Geometry check sheet. Reference: the model listing, model coordinates, mm. Round coordinates to 2 decimals unless told otherwise and drop trailing zeros. Loops run counter-clockwise (first coordinate to the right, second up) from the corner with the lowest first, then second, coordinate; pieces in that order, holes last. Notation, with made-up numbers: M 72.5,44 L 104.5,44 A13 cw 104.5,52 Z; hole C -22.5,38 d10. An arc over 180 degrees is marked long. Write item = value, one per line.
from build123d import *

# Parameters (mm, degrees)
SKETCH1_R           = 1.651
SKETCH1_R_2         = 2.286
BOSS_EXTRUDE1_DEPTH = 3.1496


with BuildPart() as part:
    # Sketch1 → Boss-Extrude1 (new body)
    with BuildSketch(Plane(origin=(0, 0, 0), x_dir=(1, 0, 0), z_dir=(0, 1, 0))):
        with BuildLine():
            Line((23.368, -25.4), (38.1, -10.668))
            Line((38.1, -10.668), (38.1, 10.668))
            Line((38.1, 10.668), (23.368, 25.4))
            Line((23.368, 25.4), (10.899655632, 25.4))
            ThreePointArc((10.899655632, 25.4), (0, 14.500344368), (-10.899655632, 25.4))
            Line((-10.899655632, 25.4), (-23.368, 25.4))
            Line((-23.368, 25.4), (-38.1, 10.668))
            Line((-38.1, 10.668), (-38.1, -10.668))
            Line((-38.1, -10.668), (-23.368, -25.4))
            Line((-23.368, -25.4), (-10.899655632, -25.4))
            ThreePointArc((-10.899655632, -25.4), (0, -14.500344368), (10.899655632, -25.4))
            Line((10.899655632, -25.4), (23.368, -25.4))
        make_face()
        with Locations(Location((-22.225, 19.05, 0), (0, 0, 270))):
            Circle(SKETCH1_R, mode=Mode.SUBTRACT)
        with Locations(Location((22.225, 19.05, 0), (0, 0, 270))):
            Circle(SKETCH1_R, mode=Mode.SUBTRACT)
        with Locations(Location((22.225, -19.05, 0), (0, 0, 270))):
            Circle(SKETCH1_R, mode=Mode.SUBTRACT)
        with Locations(Location((-22.225, -19.05, 0), (0, 0, 270))):
            Circle(SKETCH1_R, mode=Mode.SUBTRACT)
        with Locations(Location((9.271, -5.5118, 0), (0, 0, 270))):
            Circle(SKETCH1_R_2, mode=Mode.SUBTRACT)
        with Locations(Location((21.971, 5.5118, 0), (0, 0, 270))):
            Circle(SKETCH1_R_2, mode=Mode.SUBTRACT)
    extrude(amount=BOSS_EXTRUDE1_DEPTH)


solid = part.part
(1) Release check for a two-part mould opening along Z. For faces 1 (the cylindrical face through (-21.11, 1.55, -20.27)), 2 (the flat face through (-30.63, 1.55, -18.14)), 3 (the flat face through (-30.84, 1.55, 17.93)) record: released by +Z, released by -Z, zero draft, split by the parting line, or undercut.
Result set:
face_1 = undercut
face_2 = released by -Z
face_3 = released by +Z
(2) Depth check by flat-ended pin: pin 1 Ø1.5 at (x, y) = (-6, 2.5) entering from +Z; pin 2 Ø4 at (x, z) = (-22.225, 19.05) entering from -Y; pin 3 Ø2.5 at (x, z) = (9.27, 5.51) entering from +Y. Enter the tip coordinate at first touch or a pass-through.
Result set:
pin_1 = 16.84
pin_2 = 0
pin_3 = through
(3) Sectioned sample at B-B on z = -16.5. Record the cut outline in (x, y), then the cut area to 3 significant figures.
Result set:
outline = M -32.27,0 L -6.29,0 L -6.29,3.15 L -32.27,3.15 Z; M 6.29,0 L 32.27,0 L 32.27,3.15 L 6.29,3.15 Z
area = 164 mm2
(4) Sectioned sample at A-A on z = 19.05. Record the cut outline in (x, y).
Result set:
outline = M -29.72,0 L -23.88,0 L -23.88,3.15 L -29.72,3.15 Z; M -20.57,0 L -8.86,0 L -8.86,3.15 L -20.57,3.15 Z; M 8.86,0 L 20.57,0 L 20.57,3.15 L 8.86,3.15 Z; M 23.88,0 L 29.72,0 L 29.72,3.15 L 23.88,3.15 Z
(5) Sectioned sample at C-C on y = 2.5. Record the cut outline in (x, z) (3 decimals).
Result set:
outline = M -38.1,-10.668 L -23.368,-25.4 L -10.9,-25.4 A10.9 cw 10.9,-25.4 L 23.368,-25.4 L 38.1,-10.668 L 38.1,10.668 L 23.368,25.4 L 10.9,25.4 A10.9 cw -10.9,25.4 L -23.368,25.4 L -38.1,10.668 Z; hole C -22.225,-19.05 d3.302; hole C -22.225,19.05 d3.302; hole C 9.271,5.512 d4.572; hole C 21.971,-5.512 d4.572; hole C 22.225,-19.05 d3.302; hole C 22.225,19.05 d3.302
(6) Sectioned sample at D-D on x = 0. Record the cut outline in (y, z), then the cut area to 3 significant figures.
Result set:
outline = M 0,-14.5 L 3.15,-14.5 L 3.15,14.5 L 0,14.5 Z
area = 91.3 mm2
(7) Material ranges on line 1 along X through (y, z) = (2.8, 19.5); line 2 along X through (y, z) = (2.05, 18.5); line 3 along Z through (x, y) = (-22.5, 1.05), recorded low to high. Write a range as from..to.
Result set:
line_1 = -29.27..-23.81, -20.64..-9.16, 9.16..20.64, 23.81..29.27
line_2 = -30.27..-23.78, -20.67..-8.44, 8.44..20.67, 23.78..30.27
line_3 = -25.4..-20.68, -17.42..17.42, 20.68..25.4
